Job drawing, mm, ordinate dimensions from the low corner. One solid piece. Coordinates: 2 decimals unless noted, no trailing zeros. Write each loop counter-clockwise with the first axis right and the second up, starting at its lowest first coordinate (ties: lowest second). Pieces come first, ordered by that corner, then holes. Notation, with made-up numbers: (-12.5, 83.25) - (14.5, 83.25) arc R5 cw to (14.5, 90.25) - close; hole circle Ø11 at (-5, 76.25). An arc over 180 degrees is marked (long way). Put each result on its own line as item: value. Start each with the question number.
1. Saw through at B-B, the plane x = 44.5. Write the cut outline in (y, z) (1 decimal).
2. Drill centre lines: L1, parallel to Z at x = 58, y = 2.5 (1 decimal); L2, parallel to X at y = 2.15, z = 19 (1 decimal); L3, parallel to X at y = 2.2, z = 47 (1 decimal). Where is each one in solid material? Low to high. Write a range as from..to.
3. Saw through at A-A, the plane z = 34.5. Write the cut outline in (x, y) (1 decimal).
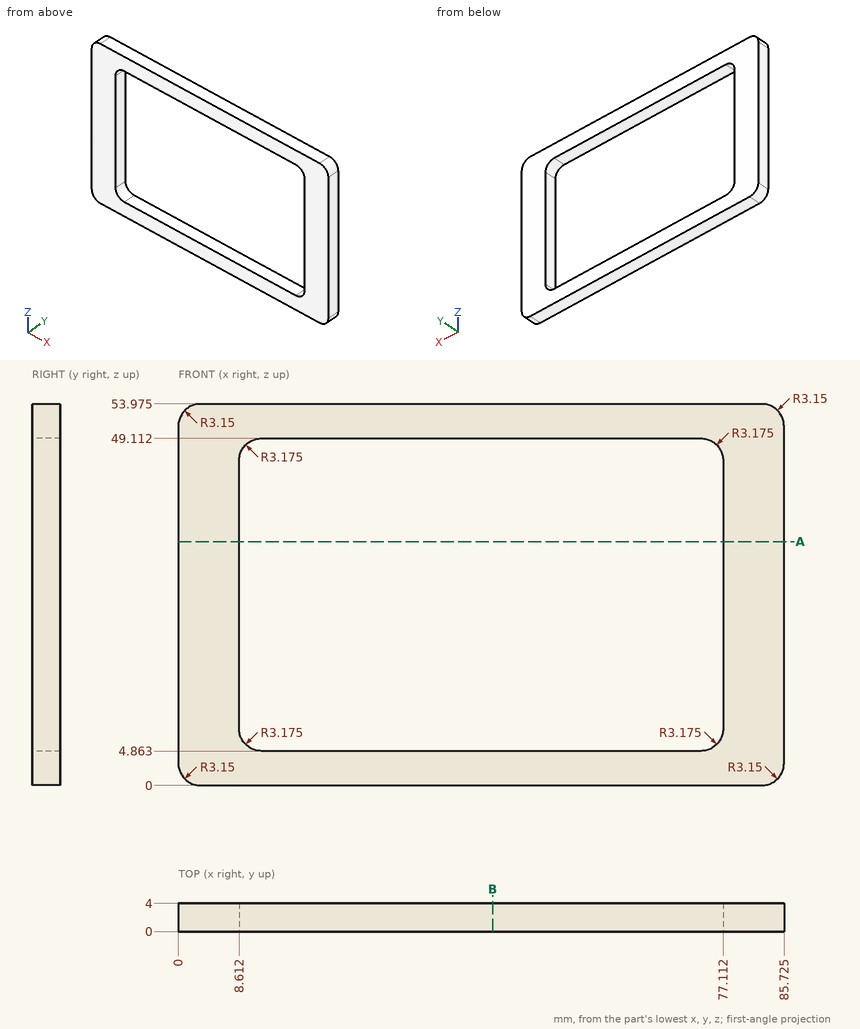
Final values:
1. outline: (0, 0) - (4, 0) - (4, 4.9) - (0, 4.9) - close; (0, 49.1) - (4, 49.1) - (4, 54) - (0, 54) - close
2. L1: z = 0..4.9, 49.1..54
2. L2: x = 0..8.6, 77.1..85.7
2. L3: x = 0..8.8, 76.9..85.7
3. outline: (0, 0) - (8.6, 0) - (8.6, 4) - (0, 4) - close; (77.1, 0) - (85.7, 0) - (85.7, 4) - (77.1, 4) - close
